The listing builds one solid part. Answer for the finished solid, in the listing's coordinates (mm). A direction names the side the tool comes from. Coordinates: 2 decimals unless noted, no trailing zeros. Order: outer loops, then holes, each group sorted by start corner. A loop starts at its lowest first (then second) coordinate and runs counter-clockwise, first axis right, second up. Notation, with made-up numbers: (75.25, -8) -> (105.25, -8) arc R31 cw to (105.25, 29) -> close; hole circle Ø9 at (21.25, -35.5). An arc over 180 degrees is marked (long way). Write each question's results on one line, items separated by ' | '. Start each with the question number.
(1) The part is cut by section C-C, the plane y = -425.5. Give the vertices of the cut face in (x, z), then the cut area to 3 significant figures.
(2) The part is cut by section A-A, the plane x = 13. Give the vertices of the cut face in (y, z), then the cut area to 3 significant figures.
(3) Straight lines are drawn through the part: L1, parallel to X at y = -157, z = 23.5; L2, parallel to Z at x = 1, y = -221. For each, find the intervals that lie inside material, in ascending order.
(4) A tool of negligible diameter and unlimited length cuts with its end or side. For faces 4 (the face through (25, -246, 29)), 5 (the face through (0, -246, -30)), from which of +Z, -Z, +X, -X, +Y, -Y can it reach the whole face along a straight path? Write none if from no direction.
(5) The part is cut by section B-B, the plane z = 6. Count the separate pieces of the cut face and the enclosed holes in it, then the cut area to 3 significant figures.
(6) The part is cut by section D-D, the plane y = -132. Give the vertices of the cut face in (x, z).
(7) Determine the mould class of faces 1 (the face through (-30, -191, -7)), 2 (the face through (-20.4, -246.5, 30)), 3 (the face through (29, -191, 0)) for opening direction Z: +Z half, -Z half, draft (parallel to the pull), parting line (faces both ways), or undercut.
```python
from build123d import *

# Parameters (mm, degrees)
F0_W     = 60
F0_H     = 60
F0_W_2   = 57.999998
F0_H_2   = 58
F1_DEPTH = 500
F2_W     = 120
F2_H     = 40
F3_DEPTH = 150
F4_W     = 40
F4_H     = 300
F5_DEPTH = 25


with BuildPart() as f1:
    # F0 (on Front) → F1 (new body)
    with BuildSketch(Plane.XZ):
        Rectangle(F0_W, F0_H)
        Rectangle(F0_W_2, F0_H_2, mode=Mode.SUBTRACT)
    extrude(amount=F1_DEPTH)

    # F2 (on face) → F3 (cut)
    with BuildSketch(Plane.YZ.offset(30)):
        with Locations((-410, 0)):
            Rectangle(F2_W, F2_H)
        with Locations((-260, 0)):
            Rectangle(F2_W, F2_H)
        with Locations((-110, 0)):
            Rectangle(F2_W, F2_H)
    extrude(amount=-F3_DEPTH, mode=Mode.SUBTRACT)

    # F4 (on face) → F5 (cut)
    with BuildSketch(Plane.XY.offset(30)):
        with Locations((0, -250)):
            Rectangle(F4_W, F4_H)
    extrude(amount=-F5_DEPTH, mode=Mode.SUBTRACT)


solid = f1.part
```
Established:
1) outline: (-30, -30) -> (30, -30) -> (30, -20) -> (29, -20) -> (29, -29) -> (-29, -29) -> (-29, -20) -> (-30, -20) -> close; (-30, 20) -> (-29, 20) -> (-29, 29) -> (29, 29) -> (29, 20) -> (30, 20) -> (30, 30) -> (-30, 30) -> close | area: 156 mm^2
2) outline: (-500, -30) -> (0, -30) -> (0, -29) -> (-500, -29) -> close; (-500, 29) -> (-400, 29) -> (-400, 30) -> (-500, 30) -> close; (-100, 29) -> (0, 29) -> (0, 30) -> (-100, 30) -> close | area: 700 mm^2
3) L1: x = -30 to -29, 29 to 30 | L2: z = -30 to -29
4) face 4: +Y, -Y | face 5: -Z, +X, -X, +Y, -Y
5) separate pieces: 8 | enclosed holes: 0 | area: 280 mm^2
6) outline: (-30, -30) -> (30, -30) -> (30, -20) -> (29, -20) -> (29, -29) -> (-29, -29) -> (-29, -20) -> (-30, -20) -> close; (-30, 20) -> (-29, 20) -> (-29, 29) -> (-20, 29) -> (-20, 30) -> (-30, 30) -> close; (20, 29) -> (29, 29) -> (29, 20) -> (30, 20) -> (30, 30) -> (20, 30) -> close
7) face 1: draft | face 2: +Z half | face 3: undercut
